from build123d import *

# Parameters (mm, degrees)
EXTRUDE1_DEPTH        = 2.9972
SKETCH2_W             = 12.7
SKETCH2_H             = 2.54
TABS_DEPTH            = 2.9972
SKETCH3_W             = 12.7
SKETCH3_H             = 3.175
SKETCH3_H_2           = 2.54
SLOTS_DEPTH           = 3.9972
SKETCH4_R             = 2.38125
HOLES_DEPTH           = 3.9972
WHEEL_CLEARANCE_DEPTH = 3.9972
FILLET1_R             = 2.54
FILLET2_R             = 4.7625
FILLET3_R             = 12.7


with BuildPart() as part:
    # Sketch1 → Extrude1 (new body)
    with BuildSketch(Plane.XY):
        Polygon((101.6, 22.225), (-101.6, 22.225), (-75.936780535, -22.225), (75.936780535, -22.225), align=None)
        Polygon((-85.102216058, 12.7), (-13.682348419, 12.7), (-28.347045256, -12.7), (-70.43751922, -12.7), align=None, mode=Mode.SUBTRACT)
        Polygon((-6.35, 12.7), (0, 12.7), (0, -12.7), (-21.014696837, -12.7), align=None, mode=Mode.SUBTRACT)
    extrude(amount=EXTRUDE1_DEPTH)

    # Sketch2 → Tabs (add, through all)
    with BuildSketch(Plane.XY.offset(2.9972)):
        with Locations((-69.85, 23.495)):
            Rectangle(SKETCH2_W, SKETCH2_H)
        with Locations((69.85, 23.495)):
            Rectangle(SKETCH2_W, SKETCH2_H)
        with Locations((0, 23.495)):
            Rectangle(SKETCH2_W, SKETCH2_H)
    extrude(amount=-TABS_DEPTH)

    # Sketch3 → Slots (cut, through all)
    with BuildSketch(Plane.XY.offset(2.9972)):
        Polygon((-94.605125878, 16.586522628), (-88.255125878, 5.588), (-85.615480447, 7.112), (-91.965480447, 18.110522628), align=None)
        with Locations((-12.7, -17.4625)):
            Rectangle(SKETCH3_W, SKETCH3_H)
        Polygon((91.965480447, 18.110522628), (85.615480447, 7.112), (88.255125878, 5.588), (94.605125878, 16.586522628), align=None)
        with Locations((63.5, -4.7625)):
            Rectangle(SKETCH3_W, SKETCH3_H_2)
    extrude(amount=-SLOTS_DEPTH, mode=Mode.SUBTRACT)

    # Sketch4 → Holes (cut, through all)
    with BuildSketch(Plane.XY.offset(2.9972)):
        with Locations((-63.5, -17.4625)):
            Circle(SKETCH4_R)
        with Locations((-44.45, -17.4625)):
            Circle(SKETCH4_R)
    extrude(amount=-HOLES_DEPTH, mode=Mode.SUBTRACT)

    # Sketch5 → Wheel Clearance (cut, through all)
    with BuildSketch(Plane.XY.offset(2.9972)):
        with BuildLine():
            Line((41.275, 19.70839808), (41.275, 1.905))
            Line((41.275, 1.905), (53.975, 1.905))
            Line((53.975, 1.905), (53.975, -6.0325))
            Line((53.975, -6.0325), (85.285524768, -6.0325))
            Line((85.285524768, -6.0325), (85.285524768, -22.225))
            Line((85.285524768, -22.225), (29.36875, -22.225))
            Line((29.36875, -22.225), (7.14375, -22.225))
            Line((7.14375, -22.225), (7.14375, -17.4625))
            ThreePointArc((7.14375, -17.4625), (16.970883995, 7.769512854), (41.275, 19.70839808))
        make_face()
    extrude(amount=-WHEEL_CLEARANCE_DEPTH, mode=Mode.SUBTRACT)

    # Fillet1
    fillet1_edges = [part.edges().sort_by_distance(p)[0] for p in [
        (-21.014696837, -12.7, 1.4986),
        (0, -12.7, 1.4986),
        (0, 12.7, 1.4986),
        (-6.35, 12.7, 1.4986),
        (-28.347045256, -12.7, 1.4986),
        (-13.682348419, 12.7, 1.4986),
        (-85.102216058, 12.7, 1.4986),
        (-70.43751922, -12.7, 1.4986),
    ]]
    fillet(fillet1_edges, radius=FILLET1_R)

    # Fillet2
    fillet2_edges = [part.edges().sort_by_distance(p)[0] for p in [
        (41.275, 19.70839808, 1.4986),
        (41.275, 1.905, 1.4986),
        (53.975, 1.905, 1.4986),
    ]]
    fillet(fillet2_edges, radius=FILLET2_R)

    # Fillet3
    fillet3_edges = [part.edges().sort_by_distance(p)[0] for p in [
        (-75.936780535, -22.225, 1.4986),
    ]]
    fillet(fillet3_edges, radius=FILLET3_R)


solid = part.part
The listing builds one solid part. Answer for the finished solid, in the listing's coordinates (mm). A direction names the side the tool comes from. Give positions to 0.01 mm unless a question says otherwise; leave off trailing zeros. Write each loop counter-clockwise with the first axis right and the second up, starting at its lowest first coordinate (ties: lowest second). Pieces come first, ordered by that corner, then holes.
1) For a pull along X with two mould halves and no side action, classify faces 4 (the face through (93.33, 7.9, 1.48)), 5 (the face through (-88.746, 12.534, 1.52)), 6 (the face through (7, 5, 0)), 7 (the face through (91.386, 11.01, 1.52)) as pulls with the +X half, pulls with the -X half, needs draft (parallel to the pull), parting line crosses it, or undercut.
2) Section C-C (x = 61.5) is taken. Write down the section's boundary in (y, z) (1 decimal), and give its area (3 significant figures).
3) Section B-B (z = 1.75) is taken. Count the separate pieces of the cut face and the enclosed holes in it, and give its area (3 significant figures).
4) Section A-A (x = -44.45) is taken. Write down the section's boundary in (y, z) (3 decimals).
5) Given P1, Ø1.5, axis at x = 91.5, z = 2, coming from the +Y side (3 decimals); P2, Ø0.8, axis at y = 23.5, z = 1.5, coming from the +X side; P3, Ø3, axis at x = -44.45, y = -17.46, coming from the -Z side, each flat-ended and moving along its own axis, determine where each tip first touches the part or whether it passes through.
6) A tool of negligible diameter and unlimited length cuts with its end or side. For faces 1 (the face through (-91.47, 11.16, 1.52)), 2 (the face through (14.817, 5.202, 1.52)), 3 (the face through (-74.87, -20.57, 1.52)), from which of +Z, -Z, +X, -X, +Y, -Y can it reach the whole face along a straight path? Write none if from no direction.
7) Find the intervals of material crossed by L1, parallel to Y at x = -44.45, z = 0.75 (3 decimals); L2, parallel to X at y = 23, z = 1.2; L3, parallel to X at y = 16.5, z = 2.2, in increasing order.
Response:
1. face 4: pulls with the +X half
1. face 5: undercut
1. face 6: needs draft
1. face 7: undercut
2. outline: (-3.5, 0) - (22.2, 0) - (22.2, 3) - (-3.5, 3) - close
2. area: 77.1 mm2
3. separate pieces: 1
3. enclosed holes: 7
3. area: 4,150 mm2
4. outline: (-22.225, 0) - (-19.844, 0) - (-19.844, 2.997) - (-22.225, 2.997) - close; (-15.081, 0) - (-12.7, 0) - (-12.7, 2.997) - (-15.081, 2.997) - close; (12.7, 0) - (22.225, 0) - (22.225, 2.997) - (12.7, 2.997) - close
5. P1: stops at y = 22.225
5. P2: stops at x = 76.2
5. P3: passes through
6. face 1: +Z, -Z
6. face 2: +Z, -Z, -Y
6. face 3: +Z, -Z, -X, -Y
7. L1: y = -22.225 to -19.844, -15.081 to -12.7, 12.7 to 22.225
7. L2: x = -76.2 to -63.5, -6.35 to 6.35, 63.5 to 76.2
7. L3: x = -98.29 to -94.56, -91.04 to 29.01, 40.63 to 91.04, 94.56 to 98.29
